The listing builds one solid part. Answer for the finished solid, in the listing's coordinates (mm). Face numbers are marked on the shaded views. A direction names the side the tool comes from. Give positions to 0.01 mm unless a question says otherwise; leave off trailing zeros. Order: outer loops, then holes, each group sorted by start corner. A loop starts at its lowest first (then second) coordinate and runs counter-clockwise, first axis right, second up. Notation, with made-up numbers: (89, 9) - (146, 9) arc R32 cw to (146, 38) - close; hole circle Ø5 at (21, -32). An arc over 180 degrees is marked (long way). Use a Markdown table: item, result. Add a question column.
1) For the marked faces 1, 2, 3 and 4, determine the directions among +Z, -Z, +X, -X, +Y, -Y from which every point of the face is accessible in a straight line to the end or side of a thin tool.
2) Flat-ended cylindrical pins translate along their axes: pin 1 (10 mm diameter, centred on x = -6, z = -0.5, fed in from -Y); pin 2 (2 mm diameter, centred on x = -3.5, y = 13, fed in from -Z); pin 3 (2 mm diameter, centred on x = 5.5, z = -2, fed in from -Y); pin 4 (10 mm diameter, centred on y = 11.5, z = 3, fed in from +X). Find the tip coordinate at first contact, or state that the pin passes through.
3) Straight lines are drawn through the part: line 1 (Z direction, x = 1.5, y = 10.75); line 2 (X direction, y = 1.25, z = 2); line 3 (Y direction, x = -3.75, z = -8.5). For each, find the intervals that lie inside material, in ascending order.
4) Find section C-C, the plane x = 0.75. Determine the outline of the cut face in (y, z), plus the area to 3 significant figures.
5) Find section A-A, the plane x = -5. Determine the outline of the cut face in (y, z), plus the area to 3 significant figures.
6) Find section B-B, the plane z = 0. Determine the outline of the cut face in (x, y).
7) Find section D-D, the plane z = 5. Determine the outline of the cut face in (x, y) (3 decimals), plus the area to 3 significant figures.
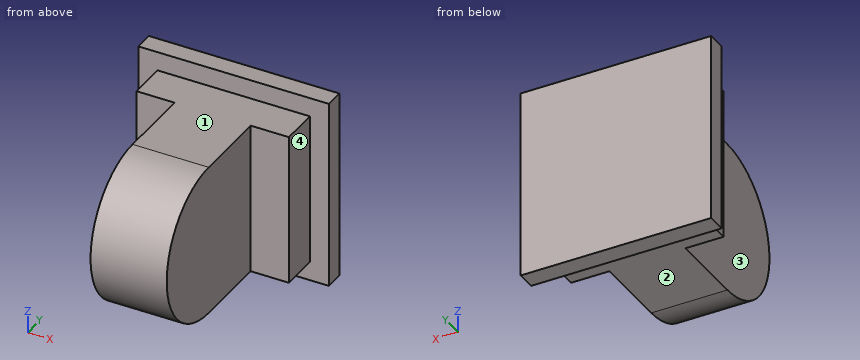
from build123d import *

# Parameters (mm, degrees)
SKETCH_1_W          = 16
SKETCH_1_H          = 16
EXTRUDE_1_DEPTH     = 20
CUT_EXTRUDE_1_DEPTH = 40
CUT_EXTRUDE_2_DEPTH = 4
CUT_EXTRUDE_3_DEPTH = 4
SKETCH_6_W          = 20
SKETCH_6_H          = 20
EXTRUDE_2_DEPTH     = 2


with BuildPart() as part:
    # 草图1 → 凸台-拉伸1 (new body)
    with BuildSketch(Plane(origin=(0, 0, 0), x_dir=(1, 0, 0), z_dir=(0, 1, 0))):
        Rectangle(SKETCH_1_W, SKETCH_1_H)
    extrude(amount=EXTRUDE_1_DEPTH)

    # 草图2 → 切除-拉伸1 (cut)
    with BuildSketch(Plane(origin=(8, 0, 0), x_dir=(0, 0, -1), z_dir=(1, 0, 0))):
        with BuildLine():
            Line((-8, 8), (-8, -6.748551072))
            Line((-8, -6.748551072), (8, -6.748551072))
            Line((8, -6.748551072), (8, 8))
            ThreePointArc((8, 8), (0, 0), (-8, 8))
        make_face()
    extrude(amount=-CUT_EXTRUDE_1_DEPTH, mode=Mode.SUBTRACT)

    # 草图4 → 切除-拉伸2 (cut)
    with BuildSketch(Plane.ZY.offset(8)):
        with BuildLine():
            Line((-8, 8), (-8, 16))
            Line((-8, 16), (8, 16))
            Line((8, 16), (8, 8))
            ThreePointArc((8, 8), (0, 0), (-8, 8))
        make_face()
    extrude(amount=-CUT_EXTRUDE_2_DEPTH, mode=Mode.SUBTRACT)

    # 草图5 → 切除-拉伸3 (cut)
    with BuildSketch(Plane(origin=(8, 0, 0), x_dir=(0, 0, -1), z_dir=(1, 0, 0))):
        with BuildLine():
            Line((-8, 8), (-8, 16))
            Line((-8, 16), (8, 16))
            Line((8, 16), (8, 8))
            ThreePointArc((8, 8), (0, 0), (-8, 8))
        make_face()
    extrude(amount=-CUT_EXTRUDE_3_DEPTH, mode=Mode.SUBTRACT)

    # 草图6 → 凸台-拉伸2 (add)
    with BuildSketch(Plane(origin=(0, 20, 0), x_dir=(1, 0, 0), z_dir=(0, 1, 0))):
        Rectangle(SKETCH_6_W, SKETCH_6_H)
    extrude(amount=EXTRUDE_2_DEPTH)


solid = part.part
The answers:
| question | item | result |
|---|---|---|
| 1 | face 1 | +Z, +X, -X, -Y |
| 1 | face 2 | -Z, +X, -X, -Y |
| 1 | face 3 | +Z, -Z, -X, -Y |
| 1 | face 4 | +Z, -Z, +X, -Y |
| 2 | pin 1 | y = 0 |
| 2 | pin 2 | z = -8 |
| 2 | pin 3 | y = 16 |
| 2 | pin 4 | x = 8 |
| 3 | line 1 | -8 to 8 |
| 3 | line 2 | -4 to 4 |
| 3 | line 3 | 20 to 22 |
| 4 | outline | (8, -8) - (20, -8) - (20, -10) - (22, -10) - (22, 10) - (20, 10) - (20, 8) - (8, 8) arc R8 ccw to start |
| 4 | area | 333 mm2 |
| 5 | outline | (16, -8) - (20, -8) - (20, -10) - (22, -10) - (22, 10) - (20, 10) - (20, 8) - (16, 8) - close |
| 5 | area | 104 mm2 |
| 6 | outline | (-10, 20) - (-8, 20) - (-8, 16) - (-4, 16) - (-4, 0) - (4, 0) - (4, 16) - (8, 16) - (8, 20) - (10, 20) - (10, 22) - (-10, 22) - close |
| 7 | outline | (-10, 20) - (-8, 20) - (-8, 16) - (-4, 16) - (-4, 1.755) - (4, 1.755) - (4, 16) - (8, 16) - (8, 20) - (10, 20) - (10, 22) - (-10, 22) - close |
| 7 | area | 218 mm2 |
